Input: part model. Units: mm. Frame: model coordinates. Face numbers are marked on the shaded views. A direction names the side the tool comes from. Give positions to 0.01 mm unless a question says otherwise; leave off trailing zeros. Loops run counter-clockwise (first coordinate to the right, second up) from the corner with the lowest first, then second, coordinate; pieces in that order, holes last. Notation, with made-up numbers: (-20, -22) -> (3, -22) arc R20 cw to (3, -7) -> close; hole circle Ø5 at (57, 88.25). An arc over 180 degrees is marked (long way). Use CSV: the item, a comma, the result in double quotes.
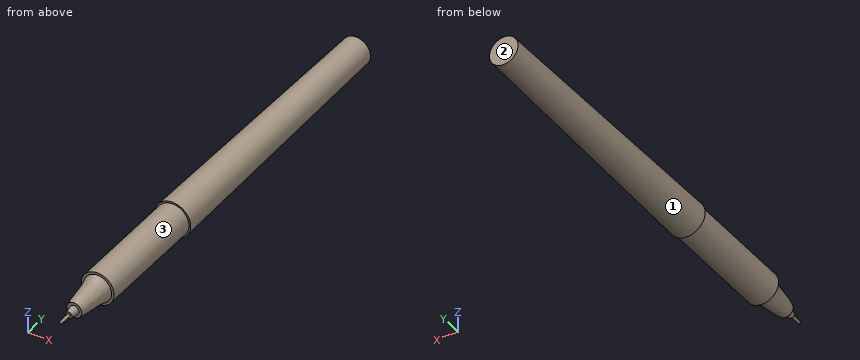
```python
from build123d import *

# Parameters (mm, degrees)
SKETCH1_R           = 4.9911
SKETCH9_R           = 3.978249141
SKETCH11_R          = 4.5466
BOSS_EXTRUDE6_DEPTH = 32.1945


with BuildPart() as part:
    # Sketch1 → Loft2 section 0
    with BuildSketch(Plane(origin=(0, 0, 0), x_dir=(1, 0, 0), z_dir=(0, 1, 0))):
        Circle(SKETCH1_R)
    # Sketch9 → Loft2 section 1
    with BuildSketch(Plane(origin=(0, 78.74, 0), x_dir=(-1, 0, 0), z_dir=(0, 1, 0))):
        Circle(SKETCH9_R)
    loft()

    # Sketch11 → Boss-Extrude6 (add)
    with BuildSketch(Plane.XZ):
        Circle(SKETCH11_R)
    extrude(amount=BOSS_EXTRUDE6_DEPTH)

    # Sketch12 → Revolve1 (revolve)
    with BuildSketch(Plane.XY):
        with BuildLine():
            Line((0, -32.1945), (3.8608, -32.1945))
            add(Edge.make_bspline(
                [(3.8608, -32.1945), (2.870537627, -34.971866769), (2.812521689, -39.84117335), (2.10185, -42.2783)],
                knots=[0, 0, 0, 0, 1, 1, 1, 1], degree=3))
            Line((2.10185, -42.2783), (0, -42.2783))
            Line((0, -42.2783), (0, -32.1945))
        make_face()
    revolve(axis=Axis((0, -1000, 0), (0, 1, 0)))

    # Sketch13 → Revolve2 (revolve)
    with BuildSketch(Plane.XY):
        Polygon((0, -42.2783), (1.31445, -42.2783), (0.92075, -44.6278), (0, -44.6278), align=None)
    revolve(axis=Axis((0, -1000, 0), (0, 1, 0)))

    # Sketch14 → Revolve3 (revolve)
    with BuildSketch(Plane.XY):
        with BuildLine():
            Line((0, -44.6278), (0.40005, -44.6278))
            Line((0.40005, -44.6278), (0.40005, -47.904449612))
            ThreePointArc((0.40005, -47.904449612), (0.283254558, -48.189563905), (0, -48.3108))
            Line((0, -48.3108), (0, -44.6278))
        make_face()
    revolve(axis=Axis((0, -1000, 0), (0, 1, 0)))


solid = part.part
```
1) Section query B-B (y = 8). Return loops of the section in (x, z).
From the geometry:
outline,"circle Ø9.78 at (0, 0)"
2) Ray query, line 1 (Y direction, x = 1.5, z = 0.75); line 2 (X direction, y = 3, z = 2); line 3 (X direction, y = 21, z = 2.75). Return the intervals inside material, ascending.
From the geometry:
line 1,"y = -42.28 to 78.74"
line 2,"x = -4.53 to 4.53"
line 3,"x = -3.84 to 3.84"
3) Contact query for flat-ended pins moving along their axis: pin 1 (3 mm diameter, centred on y = 10.5, z = 0.5, fed in from -X); pin 2 (2 mm diameter, centred on x = 0.5, z = -1, fed in from -Y); pin 3 (3 mm diameter, centred on x = 2, z = -2.5, fed in from -Y). Output: stop coordinate, or through.
From the geometry:
pin 1,"stops at x = -4.87"
pin 2,"stops at y = -48.29"
pin 3,"stops at y = -42.28"
4) Section query A-A (y = -15.5). Return loops of the section in (x, z), then the cut area to 3 significant figures.
From the geometry:
outline,"circle Ø9.09 at (0, 0)"
area,"64.9 mm^2"
5) Reachability of the marked faces 1, 2 and 3 from +Z, -Z, +X, -X, +Y, -Y: full face, straight path, thin tool, end or side. Return the list, or none.
From the geometry:
face 1,"+Y"
face 2,"+Z, -Z, +X, -X, +Y"
face 3,"-Y"
